```python
from build123d import *

# Parameters (mm, degrees)
F0_W        = 15.1496281502
F0_H        = 15.1496281502
F0_R        = 2.5
F1_DEPTH    = 25.4
F2_R        = 1.7272
F3_REACH    = 20.0358874801
F4_R        = 13.9248140751
F4_R_2      = 1.35255
F4_R_3      = 2.5
F5_DEPTH    = 4.7625
F6_T1_DEPTH = 44.3370335


# Not quite as in the source:
# - a fillet or chamfer that OpenCascade refuses, or shapes differently, is made with other operations: its cross-section is extruded or revolved along the edge and cut away or added


with BuildPart() as f1:
    # F0 (on Top) → F1 (new body)
    with BuildSketch(Plane.XY):
        Rectangle(F0_W, F0_H)
        Circle(F0_R, mode=Mode.SUBTRACT)
    extrude(amount=F1_DEPTH)

    f3_end = f1.faces().sort_by_distance((-2.5, 0, 12.7))[0]
    # F2 (on face) → F3 (cut, up to a face of the model that its end follows)
    with BuildSketch(Plane(origin=(0, 7.5748140751, 0), x_dir=(-1, 0, 0), z_dir=(0, 1, 0))):
        with Locations((0, 12.7)):
            Circle(F2_R)
    f3_long = extrude(amount=-F3_REACH, mode=Mode.PRIVATE)
    add(split(f3_long, bisect_by=f3_end, keep=Keep.ALL, mode=Mode.PRIVATE).solids().sort_by_distance((0, 7.5748140751, 12.7))[0], mode=Mode.SUBTRACT)

    # F4 (on face) → F5 (join)
    with BuildSketch(Plane(origin=(0, 0, 0), x_dir=(1, 0, 0), z_dir=(0, 0, -1))):
        Circle(F4_R)
        with Locations((-10.7498140751, 0)):
            Circle(F4_R_2, mode=Mode.SUBTRACT)
        Circle(F4_R_3, mode=Mode.SUBTRACT)
        with Locations((10.7498140751, 0)):
            Circle(F4_R_2, mode=Mode.SUBTRACT)
    extrude(amount=F5_DEPTH)

    # F6: fillet of radius 7.5748134 on 4 edges, made by hand

    # F6_s2 → F6_t1 (cut)
    with BuildSketch(Plane.XY):
        with BuildLine():
            ThreePointArc((-6.751e-07, 7.5748140751), (-5.3562025965, 5.3562025965), (-7.5748140751, 6.751e-07))
            Line((-7.5748140751, 6.751e-07), (-7.5748140751, 7.5748140751))
            Line((-7.5748140751, 7.5748140751), (-6.751e-07, 7.5748140751))
        make_face()
        with BuildLine():
            ThreePointArc((6.751e-07, 7.5748140751), (5.3562025965, 5.3562025965), (7.5748140751, 6.751e-07))
            Line((7.5748140751, 6.751e-07), (7.5748140751, 7.5748140751))
            Line((7.5748140751, 7.5748140751), (6.751e-07, 7.5748140751))
        make_face()
        with BuildLine():
            ThreePointArc((-6.751e-07, -7.5748140751), (-5.3562025965, -5.3562025965), (-7.5748140751, -6.751e-07))
            Line((-7.5748140751, -6.751e-07), (-7.5748140751, -7.5748140751))
            Line((-7.5748140751, -7.5748140751), (-6.751e-07, -7.5748140751))
        make_face()
        with BuildLine():
            ThreePointArc((6.751e-07, -7.5748140751), (5.3562025965, -5.3562025965), (7.5748140751, -6.751e-07))
            Line((7.5748140751, -6.751e-07), (7.5748140751, -7.5748140751))
            Line((7.5748140751, -7.5748140751), (6.751e-07, -7.5748140751))
        make_face()
    extrude(amount=F6_T1_DEPTH, mode=Mode.SUBTRACT)


solid = f1.part
```
Geometry: final body of the model. Coordinates: model frame, mm. A direction names the side the tool comes from. Coordinates: 2 decimals unless noted, no trailing zeros. Order: outer loops, then holes, each group sorted by start corner. A loop starts at its lowest first (then second) coordinate and runs counter-clockwise, first axis right, second up. Notation, with made-up numbers: (-4, 76) -> (21, 76) arc R30 cw to (21, 104) -> close; hole circle Ø3 at (-16.5, 85). An arc over 180 degrees is marked (long way). Write each question's results on one line, items separated by ' | '. Start each with the question number.
1) Set-up query: faces 5 (the cylindrical face through (-5.3, -5.41, 12.52)), 6 (the cylindrical face through (5.3, -5.41, 12.52)), 7 (the cylindrical face through (-5.3, 5.41, 12.52)). Return all of +Z, -Z, +X, -X, +Y, -Y with unobstructed straight access to the full face (end or side cutting, diameter ignored); none if empty.
2) Cut plane B-B, the plane x = -10.25. Output: boundary loops of the cut face in (y, z).
3) Cut plane D-D, the plane y = -5. Output: boundary loops of the cut face in (x, z), and give its area (3 significant figures).
4) Material intervals for line 1 along X through (y, z) = (0, -1.2); line 2 along Y through (x, z) = (2, 20); line 3 along Z through (x, y) = (9.25, 8), sorted ascending.
5) First-contact query: pin 1 (10 mm diameter, centred on y = -9, z = 5.5, fed in from -X); pin 2 (4 mm diameter, centred on x = 5, z = 3, fed in from +Y); pin 3 (3.5 mm diameter, centred on x = 10.75, y = 0, fed in from -Z); pin 4 (1.5 mm diameter, centred on x = -6.5, z = 9.5, fed in from +Y). Flat tips, straight axial feed; report the tip coordinate or a pass-through.
6) Mould query, pull axis Z, two halves, no side actions, for faces 1 (the flat face through (3, 0, -4.762)), 2 (the flat face through (-2, 2, 25.4)), 3 (the cylindrical face through (1.726, 4.731, 12.776)), 4 (the cylindrical face through (-0.33, -2.48, 10.53)). Classes: released by +Z, released by -Z, zero draft, split by the parting line, or undercut.
Checks:
1) face 5: +Z, -X, -Y | face 6: +Z, +X, -Y | face 7: +Z, -X, +Y
2) outline: (-9.43, -4.76) -> (-1.26, -4.76) -> (-1.26, 0) -> (-9.43, 0) -> close; (1.26, -4.76) -> (9.43, -4.76) -> (9.43, 0) -> (1.26, 0) -> close
3) outline: (-13, -4.76) -> (13, -4.76) -> (13, 0) -> (5.69, 0) -> (5.69, 25.4) -> (-5.69, 25.4) -> (-5.69, 0) -> (-13, 0) -> close | area: 413 mm^2
4) line 1: -13.92 to -12.1, -9.4 to -2.5, 2.5 to 9.4, 12.1 to 13.92 | line 2: -7.31 to -1.5, 1.5 to 7.31 | line 3: -4.76 to 0
5) pin 1: x = -6.43 | pin 2: y = 6.96 | pin 3: z = -4.76 | pin 4: y = 4.93
6) face 1: released by -Z | face 2: released by +Z | face 3: undercut | face 4: zero draft
